Geometry check sheet. Reference: the model listing, model coordinates, mm. Face numbers are marked on the shaded views. A direction names the side the tool comes from. Round coordinates to 2 decimals unless told otherwise and drop trailing zeros. Loops run counter-clockwise (first coordinate to the right, second up) from the corner with the lowest first, then second, coordinate; pieces in that order, holes last. Notation, with made-up numbers: (-20, 5.5) - (12, 5.5) arc R36 cw to (12, 40.5) - close; hole circle Ø10 at (-33, -14). An arc over 180 degrees is marked (long way). Answer in a Markdown table with one row per item. Add a question column.
```python
from build123d import *

# Parameters (mm, degrees)
F1_DEPTH = 2.54
F3_DEPTH = 2.54
F5_DEPTH = 2.54
F6_DEPTH = 2.032


with BuildPart() as f1:
    # F0 (on Top) → F1 (new body)
    with BuildSketch(Plane.XY):
        with BuildLine():
            ThreePointArc((5.5372, 0), (1.621808, 1.621808), (0, 5.5372))
            Line((0, 5.5372), (0, 11.9888))
            ThreePointArc((0, 11.9888), (1.621808, 15.904192), (5.5372, 17.526))
            Line((5.5372, 17.526), (47.2948, 17.526))
            ThreePointArc((47.2948, 17.526), (50.617543, 16.418242), (52.610808, 13.5382))
            Line((52.610808, 13.5382), (59.50739, 13.5382))
            Line((59.50739, 13.5382), (75.818647, 13.5382))
            Line((75.818647, 13.5382), (75.818647, 20.2692))
            Line((75.818647, 20.2692), (-2.5908, 20.2692))
            Line((-2.5908, 20.2692), (-2.5908, -2.7432))
            Line((-2.5908, -2.7432), (75.818647, -2.7432))
            Line((75.818647, -2.7432), (75.818647, 2.413))
            Line((75.818647, 2.413), (59.50739, 2.413))
            Line((59.50739, 2.413), (51.866447, 2.413))
            ThreePointArc((51.866447, 2.413), (49.879492, 0.640267), (47.2948, 0))
            Line((47.2948, 0), (5.5372, 0))
        make_face()
    extrude(amount=F1_DEPTH)

    # F2 (on face) → F3 (join)
    with BuildSketch(Plane.XZ.offset(2.7432)):
        Polygon((-2.5908, 0), (25.018647, 0), (22.478647, 2.54), (-2.5908, 2.54), align=None)
        Polygon((58.038647, 2.54), (55.498647, 0), (75.818647, 0), (75.818647, 2.54), align=None)
    extrude(amount=F3_DEPTH)

    # F4 (on face) → F5 (join)
    with BuildSketch(Plane(origin=(0, 20.2692, 0), x_dir=(-1, 0, 0), z_dir=(0, 1, 0))):
        Polygon((-75.818647, 0), (-55.498647, 0), (-58.038647, 2.54), (-75.818647, 2.54), align=None)
        Polygon((-22.478647, 2.54), (-25.018647, 0), (2.5908, 0), (2.5908, 2.54), align=None)
    extrude(amount=F5_DEPTH)

    # F0 (on Top) → F6 (join)
    with BuildSketch(Plane.XY):
        with BuildLine():
            ThreePointArc((59.50739, 13.5382), (65.06999, 7.9756), (59.50739, 2.413))
            Line((59.50739, 2.413), (75.818647, 2.413))
            Line((75.818647, 2.413), (75.818647, 13.5382))
            Line((75.818647, 13.5382), (59.50739, 13.5382))
        make_face()
    extrude(amount=F6_DEPTH)


solid = f1.part
```
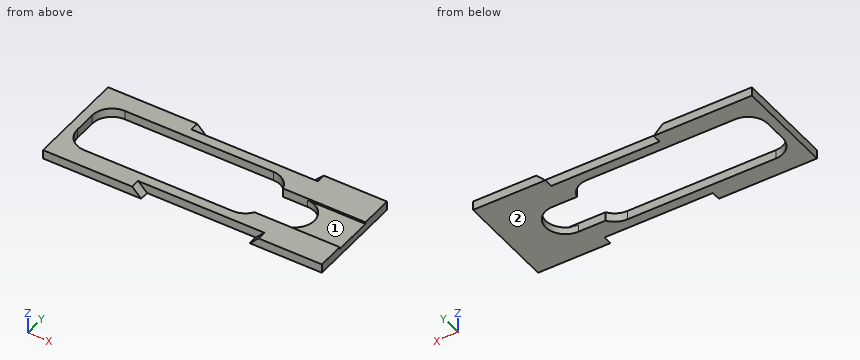
Q1. Cross-section at C-C, the plane z = 0.95. Enter the section's corners in (x, y), plus the area to 3 significant figures.
Q2. Scan lines: line 1 (Y direction, x = 27, z = 2.45); line 2 (Y direction, x = 18, z = 2.45); line 3 (X direction, y = 0.75, z = 1.9). Record each from-to range of solid material in increasing order. Write a range as from..to.
Q3. Set-up check for the marked faces 1 and 2: record each of +Z, -Z, +X, -X, +Y, -Y from which the full face is reachable in a straight line by a thin tool's end or side.
Q4. Cross-section at A-A, the plane x = 20.5. Enter the section's corners in (y, z).
Q5. Cross-section at B-B, the plane y = 8. Enter the section's corners in (x, z).
Q6. Depth check by flat-ended pin: P1, Ø0.8, axis at x = 46, z = 1, coming from the -Y side; P2, Ø0.8, axis at x = 48, z = 1, coming from the +Y side. Enter the tip coordinate at first touch or a pass-through.
Check sheet entries:
| question | item | result |
|---|---|---|
| 1 | outline | (-2.59, -5.28) - (24.07, -5.28) - (24.07, -2.74) - (56.45, -2.74) - (56.45, -5.28) - (75.82, -5.28) - (75.82, 22.81) - (56.45, 22.81) - (56.45, 20.27) - (24.07, 20.27) - (24.07, 22.81) - (-2.59, 22.81) - close; hole (0, 5.54) arc R5.54 ccw to (5.54, 0) - (47.29, 0) arc R5.54 ccw to (51.87, 2.41) - (59.51, 2.41) arc R5.56 ccw to (59.51, 13.54) - (52.61, 13.54) arc R5.54 ccw to (47.29, 17.53) - (5.54, 17.53) arc R5.54 ccw to (0, 11.99) - close |
| 1 | area | 1,010 mm² |
| 2 | line 1 | -2.74..0, 17.53..20.27 |
| 2 | line 2 | -5.28..0, 17.53..22.81 |
| 2 | line 3 | -2.59..2.75, 50.08..75.82 |
| 3 | face 1 | +Z, +X |
| 3 | face 2 | -Z, +X, -X, +Y, -Y |
| 4 | outline | (-5.28, 0) - (0, 0) - (0, 2.54) - (-5.28, 2.54) - close; (17.53, 0) - (22.81, 0) - (22.81, 2.54) - (17.53, 2.54) - close |
| 5 | outline | (-2.59, 0) - (0, 0) - (0, 2.54) - (-2.59, 2.54) - close; (65.07, 0) - (75.82, 0) - (75.82, 2.03) - (65.07, 2.03) - close |
| 6 | P1 | y = -2.74 |
| 6 | P2 | y = 20.27 |
